from build123d import *

# Parameters (mm, degrees)
SKETCH1_W                                        = 75
SKETCH1_H                                        = 60
BOSS_EXTRUDE1_DEPTH                              = 12.7
CSK_FOR_1_4_FLAT_HEAD_MACHINE_SCREW1_D           = 6.5278
CSK_FOR_1_4_FLAT_HEAD_MACHINE_SCREW1_CSINK_D     = 12.8778
CSK_FOR_1_4_FLAT_HEAD_MACHINE_SCREW1_CSINK_ANGLE = 82
FILLET1_R                                        = 2


with BuildPart() as part:
    # Sketch1 → Boss-Extrude1 (new body)
    with BuildSketch(Plane.XY):
        with Locations((37.5, -30)):
            Rectangle(SKETCH1_W, SKETCH1_H)
        Polygon((21.625, -3.367091904), (21.625, -16.067091904), (53.375, -16.067091904), (53.375, -3.367091904), (37.5, -3.367091904), align=None, mode=Mode.SUBTRACT)
    extrude(amount=BOSS_EXTRUDE1_DEPTH)

    # CSK for 1/4 Flat Head Machine Screw1 (through all)
    with Locations(Plane(origin=(0, 0, 0), x_dir=(-1, 0, 0), z_dir=(0, 0, -1))):
        with Locations((-67.49, -9.717091904), (-7.51, -9.717091904)):
            CounterSinkHole(CSK_FOR_1_4_FLAT_HEAD_MACHINE_SCREW1_D / 2, CSK_FOR_1_4_FLAT_HEAD_MACHINE_SCREW1_CSINK_D / 2, counter_sink_angle=CSK_FOR_1_4_FLAT_HEAD_MACHINE_SCREW1_CSINK_ANGLE)

    # Fillet1
    fillet1_edges = [part.edges().sort_by_distance(p)[0] for p in [
        (0, 0, 6.35),
        (75, 0, 6.35),
        (75, -60, 6.35),
        (0, -60, 6.35),
    ]]
    fillet(fillet1_edges, radius=FILLET1_R)


solid = part.part
The model under review builds one solid part; all positions refer to its coordinate system, in mm. A direction names the side the tool comes from. Give positions to 0.01 mm unless a question says otherwise; leave off trailing zeros. Order: outer loops, then holes, each group sorted by start corner. A loop starts at its lowest first (then second) coordinate and runs counter-clockwise, first axis right, second up. Notation, with made-up numbers: M 64.25,68 L 94.25,68 A10 cw 94.25,78 Z; hole C -18.75,67 d7. An arc over 180 degrees is marked long. One line per question, with ' | ' between items. Start each with the question number.
1) Wall thickness on L1, parallel to X at y = -10, z = 6 (3 decimals); L2, parallel to Y at x = 42, z = 9; L3, parallel to X at y = -7, z = 9.25 (3 decimals): over which ranges is each line inside the solid? List them lowest first. Write a range as from..to.
2) Mouldability with a two-part tool opening along X and no side actions: class faces 3 (the face through (37, -3.367, 6)), 4 (the face through (74.43, -0.6, 6.44)), 5 (the face through (21.625, -10, 6)), 6 (the face through (37, -60, 6)) as pulls with the +X half, pulls with the -X half, needs draft (parallel to the pull), parting line crosses it, or undercut.
3) Consider section B-B, the plane z = 10. Give the boundary of the cut face in (x, y) (3 decimals).
4) Consider section D-D, the plane z = 1.75. Give the boundary of the cut face in (x, y) (3 decimals), then the cut area to 3 significant figures.
5) Consider section A-A, the plane x = 22.5. Give the boundary of the cut face in (y, z), then the cut area to 3 significant figures.
6) For faces 1 (the face through (37, 0, 6)), 2 (the face through (53.375, -10, 6)), list the 3-axis set-ups (+Z, -Z, +X, -X, +Y, -Y) from which the entire face can be reached by the end or side of a thin tool; tool diameter is ignored.
7) Consider section C-C, the plane x = 67.49. Give the boundary of the cut face in (y, z), then the cut area to 4 significant figures.
Found:
1) L1: x = 0..4.258, 10.762..21.625, 53.375..64.238, 70.742..75 | L2: y = -60..-16.07, -3.37..0 | L3: x = 0..5.702, 9.318..21.625, 53.375..65.682, 69.298..75
2) face 3: undercut | face 4: pulls with the +X half | face 5: undercut | face 6: needs draft
3) outline: M 0,-58 A2 ccw 2,-60 L 73,-60 A2 ccw 75,-58 L 75,-2 A2 ccw 73,0 L 2,0 A2 ccw 0,-2 Z; hole C 7.51,-9.717 d6.528; hole M 21.625,-16.067 L 53.375,-16.067 L 53.375,-3.367 L 21.625,-3.367 Z; hole C 67.49,-9.717 d6.528
4) outline: M 0,-58 A2 ccw 2,-60 L 73,-60 A2 ccw 75,-58 L 75,-2 A2 ccw 73,0 L 2,0 A2 ccw 0,-2 Z; hole C 7.51,-9.717 d9.835; hole M 21.625,-16.067 L 53.375,-16.067 L 53.375,-3.367 L 21.625,-3.367 Z; hole C 67.49,-9.717 d9.835 | area: 3,940 mm²
5) outline: M -60,0 L -16.07,0 L -16.07,12.7 L -60,12.7 Z; M -3.37,0 L 0,0 L 0,12.7 L -3.37,12.7 Z | area: 601 mm²
6) face 1: +Z, -Z, +X, -X, +Y | face 2: +Z, -Z
7) outline: M -60,0 L -16.16,0 L -12.98,3.65 L -12.98,12.7 L -60,12.7 Z; M -6.45,3.65 L -3.28,0 L 0,0 L 0,12.7 L -6.45,12.7 Z | area: 667.5 mm²
